Can you work these out from the model? Positions are in its coordinate system, mm. Face numbers are marked on the shaded views. Give positions to 0.01 mm unless a question says otherwise; leave off trailing zeros. Loops run counter-clockwise (first coordinate to the right, second up) from the corner with the lowest first, then second, coordinate; pieces in that order, holes last. Notation, with made-up numbers: (46.25, -4.75) - (103.25, -4.75) arc R29 cw to (103.25, 28.25) - close; hole circle Ø2 at (18.5, 23). An arc over 180 degrees is marked (long way). Answer as a JSON object with one key per item and string values.
```python
from build123d import *

# Parameters (mm, degrees)
BOSS_EXTRUDE1_OUTLINE_R   = 55
BOSS_EXTRUDE1_OUTLINE_R_2 = 1.6
BOSS_EXTRUDE1_DEPTH       = 5
SKETCH2_R                 = 50
BOSS_EXTRUDE2_DEPTH       = 20
SKETCH3_R                 = 40
CUT_EXTRUDE1_DEPTH        = 82.700673192


# Read off the part's stored shape, not the designer's step: Boss-Extrude1
with BuildPart() as part:
    # Boss-Extrude1 outline → Boss-Extrude1 (new body)
    with BuildSketch(Plane(origin=(0, 0, 0), x_dir=(1, 0, 0), z_dir=(0, 1, 0))):
        Circle(BOSS_EXTRUDE1_OUTLINE_R)
        with Locations((-37.123106012, -37.123106012)):
            Circle(BOSS_EXTRUDE1_OUTLINE_R_2, mode=Mode.SUBTRACT)
        with Locations((0, -52.5)):
            Circle(BOSS_EXTRUDE1_OUTLINE_R_2, mode=Mode.SUBTRACT)
        with Locations((37.123106012, -37.123106012)):
            Circle(BOSS_EXTRUDE1_OUTLINE_R_2, mode=Mode.SUBTRACT)
        with Locations((-52.5, 0)):
            Circle(BOSS_EXTRUDE1_OUTLINE_R_2, mode=Mode.SUBTRACT)
        with Locations((-37.123106012, 37.123106012)):
            Circle(BOSS_EXTRUDE1_OUTLINE_R_2, mode=Mode.SUBTRACT)
        with Locations((52.5, 0)):
            Circle(BOSS_EXTRUDE1_OUTLINE_R_2, mode=Mode.SUBTRACT)
        with Locations((0, 52.5)):
            Circle(BOSS_EXTRUDE1_OUTLINE_R_2, mode=Mode.SUBTRACT)
        with Locations((37.123106012, 37.123106012)):
            Circle(BOSS_EXTRUDE1_OUTLINE_R_2, mode=Mode.SUBTRACT)
    extrude(amount=BOSS_EXTRUDE1_DEPTH)

    # Sketch2 → Boss-Extrude2 (add)
    with BuildSketch(Plane(origin=(0, 5, 0), x_dir=(1, 0, 0), z_dir=(0, 1, 0))):
        with Locations(Location((0, 0, 0), (0, 0, 270))):
            Circle(SKETCH2_R)
    extrude(amount=BOSS_EXTRUDE2_DEPTH)

    # Sketch3 → Cut-Extrude1 (cut, through all)
    with BuildSketch(Plane(origin=(0, 25, 0), x_dir=(1, 0, 0), z_dir=(0, 1, 0))):
        with Locations(Location((0, 0, 0), (0, 0, 270))):
            Circle(SKETCH3_R)
    extrude(amount=-CUT_EXTRUDE1_DEPTH, mode=Mode.SUBTRACT)


solid = part.part
```
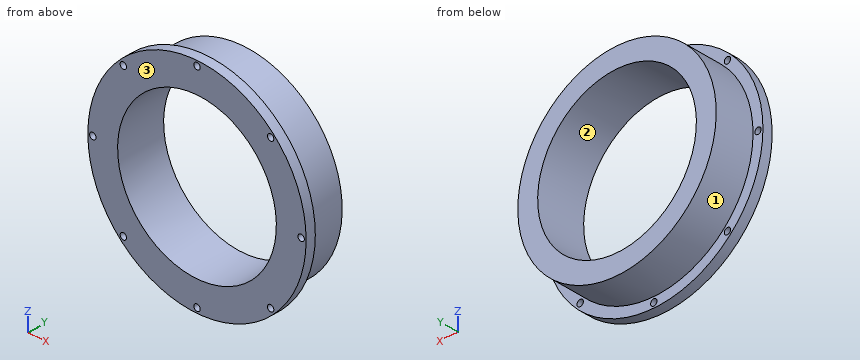
1) I'm going to push flat-ended pins straight in: P1, Ø8, axis at x = -10.5, y = 16, coming from the +Z side; P2, Ø3, axis at x = -39.5, z = -22, coming from the -Y side; P3, Ø1, axis at y = 19.5, z = -14, coming from the +X side; P4, Ø1, axis at x = -3.5, y = 19, coming from the +Z side. Where does each tip first touch, or does it pass through?
Check sheet entries:
{"P1": "z = 49.58", "P2": "y = 0", "P3": "x = 48.14", "P4": "z = 49.91"}
2) If we mould it in two halves opening along X, with no side actions, what happens to the marked faces 1, 2 and 3? For each: released by +X, released by -X, zero draft, split by the parting line, or undercut.
Check sheet entries:
{"face 1": "split by the parting line", "face 2": "undercut", "face 3": "zero draft"}
3) Imagine slicing it at C-C on x = -32. Write out the boundary of the cut face in (y, z), and give its area (3 significant figures).
Check sheet entries:
{"outline": "(0, -44.73) - (5, -44.73) - (5, -38.42) - (25, -38.42) - (25, -24) - (0, -24) - close; (0, 24) - (25, 24) - (25, 38.42) - (5, 38.42) - (5, 44.73) - (0, 44.73) - close", "area": "784 mm2"}
4) Imagine slicing it at B-B on z = 0. Write out the boundary of the cut face in (x, y).
Check sheet entries:
{"outline": "(-55, 0) - (-54.1, 0) - (-54.1, 5) - (-55, 5) - close; (-50.9, 0) - (-40, 0) - (-40, 25) - (-50, 25) - (-50, 5) - (-50.9, 5) - close; (40, 0) - (50.9, 0) - (50.9, 5) - (50, 5) - (50, 25) - (40, 25) - close; (54.1, 0) - (55, 0) - (55, 5) - (54.1, 5) - close"}
5) I need wall thicknesses on L1, parallel to Z at x = 10, y = 3.25; L2, parallel to X at y = 18.25, z = 0; L3, parallel to Z at x = -23, y = 22. Which ranges of each line are inside material? Lowest first, please.
Check sheet entries:
{"L1": "-54.08 to -38.73, 38.73 to 54.08", "L2": "-50 to -40, 40 to 50", "L3": "-44.4 to -32.73, 32.73 to 44.4"}
6) Imagine slicing it at D-D on z = 19. Write out the boundary of the cut face in (x, y), and give its area (3 significant figures).
Check sheet entries:
{"outline": "(-51.61, 0) - (-35.2, 0) - (-35.2, 25) - (-46.25, 25) - (-46.25, 5) - (-51.61, 5) - close; (35.2, 0) - (51.61, 0) - (51.61, 5) - (46.25, 5) - (46.25, 25) - (35.2, 25) - close", "area": "606 mm2"}
7) Imagine slicing it at A-A on x = 0. Write out the boundary of the cut face in (y, z).
Check sheet entries:
{"outline": "(0, -55) - (5, -55) - (5, -54.1) - (0, -54.1) - close; (0, -50.9) - (5, -50.9) - (5, -50) - (25, -50) - (25, -40) - (0, -40) - close; (0, 40) - (25, 40) - (25, 50) - (5, 50) - (5, 50.9) - (0, 50.9) - close; (0, 54.1) - (5, 54.1) - (5, 55) - (0, 55) - close"}
